Autodesk Inventor part; units mm, degrees
ref_plane "YZ Plane" through (0, 0, 0) normal (1, 0, 0) x (0, 1, 0)
ref_plane "XZ Plane" through (0, 0, 0) normal (0, 1, 0) x (-1, 0, 0)
ref_plane "XY Plane" through (0, 0, 0) normal (0, 0, 1) x (1, 0, 0)
sketch "Sketch1" plane through (0, 0, 0) normal (0, 1, 0) x (-1, 0, 0)
  circle A0 centre (-15.2763, 11.7192) radius 2.1844
  circle A1 centre (46.1983, -4.1823) radius 2.1844
  circle A2 centre (-0.2854, 25.8488) radius 2.1844
  circle A3 centre (17.6488, 27.2646) radius 2.1844
  circle A4 centre (23.5893, -10.3689) radius 2.1844
  circle A5 centre (-38.3261, 27.9733) radius 2.1844
  arc A6 (-38.2458, 34.3228) -> (-41.6694, 22.5746) centre (-38.3261, 27.9733) ccw
  arc A7 (20.246, -15.7676) -> (25.2652, -16.4937) centre (23.5893, -10.3689) ccw
  line L0 (-41.6694, 22.5746) -> (20.246, -15.7676)
  arc A8 (22.3503, 31.5329) -> (17.7292, 33.6141) centre (17.6488, 27.2646) ccw
  line L1 (17.7292, 33.6141) -> (-38.2458, 34.3228)
  arc A9 (47.8742, -10.3072) -> (50.8998, 0.086) centre (46.1983, -4.1823) ccw
  line L2 (50.8998, 0.086) -> (22.3503, 31.5329)
  line L3 (47.8742, -10.3072) -> (25.2652, -16.4937)
  point P0 (0, 0)
  point P1 (21.7554, 32.108)
  point P2 (24.1332, -16.6956)
extrude "Extrusion1" add sketch "Sketch1" along normal blind 1.5875
properties part number "newsidepolytest"
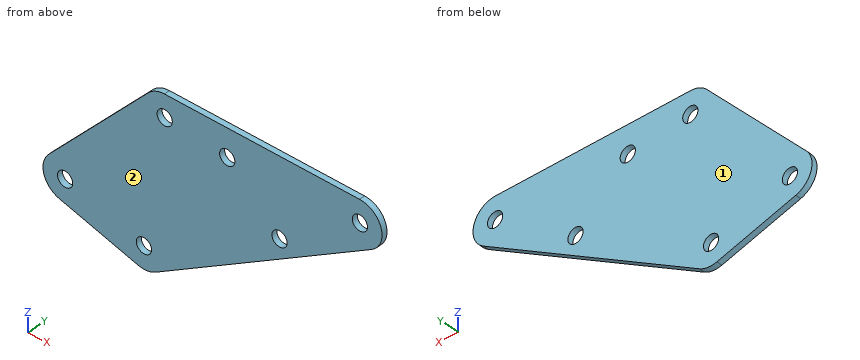
The listing builds one solid part. Answer for the finished solid, in the listing's coordinates (mm). Face numbers are marked on the shaded views. Coordinates: 2 decimals unless noted, no trailing zeros. Write each loop counter-clockwise with the first axis right and the second up, starting at its lowest first coordinate (ties: lowest second). Pieces come first, ordered by that corner, then holes. Notation, with made-up numbers: M 20,11 L 38,11 A18 cw 38,44 Z; hole C 85,23.25 d6. An arc over 180 degrees is marked long. Use one line per item in the form item = value.
Item 1: The mould has two halves that part along Y. Classify the marked faces 1 and 2: released by +Y, released by -Y, zero draft, split by the parting line, or undercut.
Model answer:
face_1 = released by +Y
face_2 = released by -Y
Item 2: Find section B-B, the plane x = -32. Give the vertices of the cut face in (y, z).
Model answer:
outline = M 0,-14.65 L 1.59,-14.65 L 1.59,20.9 L 0,20.9 Z
Item 3: Given P1, Ø5.5, axis at x = -46.2, z = -4.18, coming from the -Y side, flat-ended and moving along its own axis, determine where the tip first touches the part or whether it passes through.
Model answer:
P1 = 0
Item 4: Find the intervals of material crossed by probe 1 along X at (y, z) = (0.9, 29); probe 2 along X at (y, z) = (1.2, 27.5); probe 3 along X at (y, z) = (0.9, 12.5), in increasing order.
Model answer:
probe_1 = -24.65 to -18.98, -16.32 to 36.4, 40.25 to 44.59
probe_2 = -26.01 to -19.82, -15.48 to -1.14, 1.72 to 36.19, 40.46 to 44.66
probe_3 = -39.63 to 13.24, 17.32 to 25.4
Item 5: Find section A-A, the plane y = 0.9. Give the vertices of the cut face in (x, z), plus the area to 3 significant figures.
Model answer:
outline = M -50.9,0.09 A6.35 ccw -47.87,-10.31 L -25.27,-16.49 A6.35 ccw -20.25,-15.77 L 41.67,22.57 A6.35 ccw 38.25,34.32 L -17.73,33.61 A6.35 ccw -22.35,31.53 Z; hole C -46.2,-4.18 d4.37; hole C -23.59,-10.37 d4.37; hole C -17.65,27.26 d4.37; hole C 0.29,25.85 d4.37; hole C 15.28,11.72 d4.37; hole C 38.33,27.97 d4.37
area = 2,770 mm2
Item 6: Find section C-C, the plane z = 7.5. Give the vertices of the cut face in (x, y), plus the area to 3 significant figures.
Model answer:
outline = M -44.17,0 L 17.33,0 L 17.33,1.59 L -44.17,1.59 Z
area = 97.6 mm2
